Design review of the part built by this model. Coordinates are the model's own, in mm. Coordinates: 2 decimals unless noted, no trailing zeros. Order: outer loops, then holes, each group sorted by start corner. A loop starts at its lowest first (then second) coordinate and runs counter-clockwise, first axis right, second up. Notation, with made-up numbers: (-13.5, 34.25) -> (12.5, 34.25) arc R16 ccw to (12.5, 51.25) -> close; hole circle Ø10 at (20.5, 51). An arc over 180 degrees is marked (long way). Write item = value, one per line.
```python
from build123d import *

# Parameters (mm, degrees)
ESQUISSE1_W             = 49
ESQUISSE1_H             = 283
ESQUISSE1_R             = 1.5
BOSS_EXTRU_1_DEPTH      = 2
ESQUISSE2_W             = 42.8
ESQUISSE2_H             = 18.6
ESQUISSE2_W_2           = 4
ESQUISSE2_H_2           = 17
BOSS_EXTRU_2_DEPTH      = 16
ESQUISSE3_R             = 1.5
ENL_V_MAT_EXTRU_1_DEPTH = 16


with BuildPart() as part:
    # Esquisse1 → Boss.-Extru.1 (new body)
    with BuildSketch(Plane(origin=(0, 0, 0), x_dir=(1, 0, 0), z_dir=(0, 1, 0))):
        Rectangle(ESQUISSE1_W, ESQUISSE1_H)
        with Locations((12.65, 74.2)):
            Circle(ESQUISSE1_R, mode=Mode.SUBTRACT)
        with Locations((-17.35, 74.2)):
            Circle(ESQUISSE1_R, mode=Mode.SUBTRACT)
        with Locations((-17.35, 44.2)):
            Circle(ESQUISSE1_R, mode=Mode.SUBTRACT)
        with Locations((-17.35, 14.2)):
            Circle(ESQUISSE1_R, mode=Mode.SUBTRACT)
        with Locations((-17.35, -15.8)):
            Circle(ESQUISSE1_R, mode=Mode.SUBTRACT)
        with Locations((-17.35, -45.8)):
            Circle(ESQUISSE1_R, mode=Mode.SUBTRACT)
        with Locations((-17.35, -75.8)):
            Circle(ESQUISSE1_R, mode=Mode.SUBTRACT)
        with Locations((-17.35, -105.8)):
            Circle(ESQUISSE1_R, mode=Mode.SUBTRACT)
        with Locations((-17.35, -135.8)):
            Circle(ESQUISSE1_R, mode=Mode.SUBTRACT)
        with Locations((12.65, 44.2)):
            Circle(ESQUISSE1_R, mode=Mode.SUBTRACT)
        with Locations((12.65, 14.2)):
            Circle(ESQUISSE1_R, mode=Mode.SUBTRACT)
        with Locations((12.65, -15.8)):
            Circle(ESQUISSE1_R, mode=Mode.SUBTRACT)
        with Locations((12.65, -45.8)):
            Circle(ESQUISSE1_R, mode=Mode.SUBTRACT)
        with Locations((12.65, -75.8)):
            Circle(ESQUISSE1_R, mode=Mode.SUBTRACT)
        with Locations((12.65, -105.8)):
            Circle(ESQUISSE1_R, mode=Mode.SUBTRACT)
        with Locations((12.65, -135.8)):
            Circle(ESQUISSE1_R, mode=Mode.SUBTRACT)
    extrude(amount=BOSS_EXTRU_1_DEPTH)

    # Esquisse2 → Boss.-Extru.2 (add)
    with BuildSketch(Plane.XZ):
        with Locations((3.1, -106.8)):
            Rectangle(ESQUISSE2_W, ESQUISSE2_H)
        with Locations((-21.1, -133)):
            Rectangle(ESQUISSE2_W_2, ESQUISSE2_H_2)
        with Locations((22.5, -133)):
            Rectangle(ESQUISSE2_W_2, ESQUISSE2_H_2)
    extrude(amount=BOSS_EXTRU_2_DEPTH)

    # Esquisse3 → Enlèv. mat.-Extru.1 (cut)
    with BuildSketch(Plane.XZ):
        with Locations((-0.5, -134.5)):
            Circle(ESQUISSE3_R)
    extrude(amount=-ENL_V_MAT_EXTRU_1_DEPTH, mode=Mode.SUBTRACT)


solid = part.part
```
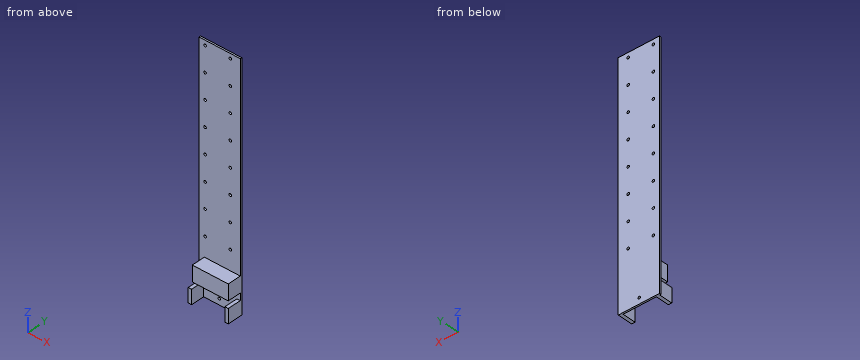
(1) We need section B-B (z = -86). Write out the cut boundary in (x, y).
Report:
outline = (-24.5, 0) -> (24.5, 0) -> (24.5, 2) -> (-24.5, 2) -> close
(2) For L1, parallel to X at y = 1.2, z = 105.8; L2, parallel to Z at x = 22.5, y = -1.25; L3, parallel to Y at x = -20.5, z = -104, list the stretches that pass through material, from the lowest coordinate up.
Report:
L1 = -24.5 to -18.85, -15.85 to 11.15, 14.15 to 24.5
L2 = -141.5 to -124.5, -116.1 to -97.5
L3 = 0 to 2
(3) We need section A-A (y = -9.5). Write out the cut boundary in (x, z).
Report:
outline = (-23.1, -141.5) -> (-19.1, -141.5) -> (-19.1, -124.5) -> (-23.1, -124.5) -> close; (-18.3, -116.1) -> (24.5, -116.1) -> (24.5, -97.5) -> (-18.3, -97.5) -> close; (20.5, -141.5) -> (24.5, -141.5) -> (24.5, -124.5) -> (20.5, -124.5) -> close
(4) Insertion check: pin 1 (3.5 mm diameter, centred on x = -17.35, z = 75.8, fed in from -Y); pin 2 (5 mm diameter, centred on x = 11, y = -8.5, fed in from +Z); pin 3 (3 mm diameter, centred on x = -8, y = -11.5, fed in from -Z). Each pin has a flat end and moves straight along its axis. Give the tip position at first contact, or say it passes through.
Report:
pin_1 = 0
pin_2 = -97.5
pin_3 = -116.1
